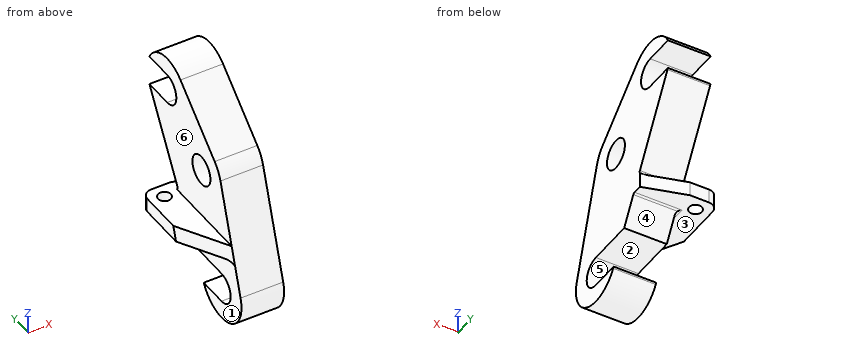
from build123d import *

# Parameters (mm, degrees)
SKETCH1_R                       = 3.15
BOSS_EXTRUDE1_DEPTH             = 9
BOSS_EXTRUDE2_DEPTH             = 6
BOSS_EXTRUDE2_DIRECTION_2_REACH = 244.867
SKETCH3_R                       = 1.35
CUT_EXTRUDE1_DEPTH              = 242.551945874
CHAMFER1_SIZE                   = 6
CHAMFER1_SIZE_2                 = 10
CHAMFER2_SIZE                   = 2.6
CHAMFER2_SIZE2                  = 9
FILLET1_R                       = 2
FILLET2_R                       = 0.5
FILLET3_R                       = 0.5
FILLET4_R                       = 1


with BuildPart() as part:
    # Sketch1 → Boss-Extrude1 (new body)
    with BuildSketch(Plane(origin=(9, 0, 0), x_dir=(0, 0, -1), z_dir=(1, 0, 0))):
        with BuildLine():
            Line((3.523521467, 220.170630859), (3.223774703, 220.343673039))
            Line((3.223774703, 220.343673039), (3.223774703, 214.108306834))
            ThreePointArc((3.223774703, 214.108306834), (0.023774703, 210.908306834), (-3.176225297, 214.108306834))
            Line((-3.176225297, 214.108306834), (-3.176225297, 224.038358312))
            Line((-3.176225297, 224.038358312), (-29.477274378, 239.221811231))
            ThreePointArc((-29.477274378, 239.221811231), (-29.626151265, 239.305353383), (-29.777021142, 239.385240172))
            Line((-29.777021142, 239.385240172), (-29.777021142, 233.159487206))
            ThreePointArc((-29.777021142, 233.159487206), (-32.977021142, 229.959487206), (-36.177021142, 233.159487206))
            Line((-36.177021142, 233.159487206), (-36.177021142, 239.385240172))
            ThreePointArc((-36.177021142, 239.385240172), (-39.85809233, 234.444344903), (-38.208056262, 228.508006627))
            Line((-38.208056262, 228.508006627), (-27.537554982, 216.508006627))
            ThreePointArc((-27.537554982, 216.508006627), (-26.112876869, 215.284825825), (-24.414305812, 214.484366354))
            Line((-24.414305812, 214.484366354), (-2.084011246, 207.433185982))
            ThreePointArc((-2.084011246, 207.433185982), (6.430412997, 211.287848401), (3.523521467, 220.170630859))
        make_face()
        with Locations(Location((-22.306519862, 221.159487206, 0), (0, 0, 180))):
            Circle(SKETCH1_R, mode=Mode.SUBTRACT)
    extrude(amount=-BOSS_EXTRUDE1_DEPTH)

    # Sketch2 → Boss-Extrude2 (add)
    with BuildSketch(Plane.ZY):
        Polygon((8.976225297, 232.108306834), (11.976225297, 232.108306834), (11.976225297, 210.556825276), (8.976225297, 209.609522899), align=None)
    extrude(amount=BOSS_EXTRUDE2_DEPTH)

    # Boss-Extrude2 direction 2: up to this face of the body (flat: up to its plane)
    boss_extrude2_direction_2_end = Plane(part.part.faces().sort_by_distance((9, 222.248813277, 17.342130355))[0])
    # Sketch2 → Boss-Extrude2 direction 2 (add, up to the picked face)
    with BuildSketch(Plane.ZY, mode=Mode.PRIVATE) as boss_extrude2_direction_2_sk1:
        Polygon((8.976225297, 232.108306834), (11.976225297, 232.108306834), (11.976225297, 210.556825276), (8.976225297, 209.609522899), align=None)
    boss_extrude2_direction_2_tool1 = split(extrude(boss_extrude2_direction_2_sk1.sketch, amount=-BOSS_EXTRUDE2_DIRECTION_2_REACH, mode=Mode.PRIVATE), bisect_by=boss_extrude2_direction_2_end, keep=Keep.BOTH, mode=Mode.PRIVATE)
    add(boss_extrude2_direction_2_tool1.solids().sort_by(Axis((0, 221.094043, 10.465473), (1, 0, 0)))[0])

    # Sketch3 → Cut-Extrude1 (cut, through all)
    with BuildSketch(Plane(origin=(0, 0, 8.976225297), x_dir=(-1, 0, 0), z_dir=(0, 0, -1))):
        with Locations(Location((3, 229.108306834, 0), (0, 0, 90))):
            Circle(SKETCH3_R)
    extrude(amount=-CUT_EXTRUDE1_DEPTH, mode=Mode.SUBTRACT)

    # Chamfer1
    # the kernel refuses this chamfer: 10, 6 mm, written as the material it takes off along each edge
    with BuildSketch(Plane(origin=(-6, 218.344374993, 36.638518695), x_dir=(0.9984760801092615, -0.05262494307091041, 0.016617244549774337), z_dir=(0, -0.3011122785042559, -0.9535886931659664))) as chamfer1_piece_1:
        Polygon((CHAMFER1_SIZE * 0.998476080109, -CHAMFER1_SIZE * 0.0551862070598), (-CHAMFER1_SIZE_2 * 0.0551862070598, -CHAMFER1_SIZE_2 * 0.998476080109), (0, 0), align=None)
    extrude(amount=54.8712324, mode=Mode.SUBTRACT)

    # Chamfer2
    chamfer2_edges = [part.edges().sort_by_distance(p)[0] for p in [
        (9, 232.108306834, 10.476225297),
    ]]
    chamfer2_side = [part.faces().sort_by_distance(p)[0] for p in [
        (9, 222.390108053, 17.217310228),
    ]]
    chamfer(chamfer2_edges, length=CHAMFER2_SIZE, length2=CHAMFER2_SIZE2, reference=chamfer2_side[0])

    # Fillet1
    fillet1_edges = [part.edges().sort_by_distance(p)[0] for p in [
        (-6, 232.108306834, 10.476225297),
    ]]
    fillet(fillet1_edges, radius=FILLET1_R)

    # Fillet2
    fillet2_edges = [part.edges().sort_by_distance(p)[0] for p in [
        (4.5, 227.38666684, 8.976225297),
    ]]
    fillet(fillet2_edges, radius=FILLET2_R)

    # Fillet3
    fillet3_edges = [part.edges().sort_by_distance(p)[0] for p in [
        (4.5, 229.118550561, 11.976225297),
    ]]
    fillet(fillet3_edges, radius=FILLET3_R)

    # Fillet4
    fillet4_edges = [part.edges().sort_by_distance(p)[0] for p in [
        (0, 218.642439399, 8.976225297),
    ]]
    fillet(fillet4_edges, radius=FILLET4_R)


solid = part.part
Geometry: final body of the model. Coordinates: model frame, mm. Face numbers are marked on the shaded views. A direction names the side the tool comes from. Give positions to 0.01 mm unless a question says otherwise; leave off trailing zeros. Order: outer loops, then holes, each group sorted by start corner. A loop starts at its lowest first (then second) coordinate and runs counter-clockwise, first axis right, second up. Notation, with made-up numbers: (-27, -1) -> (4, -1) arc R22 cw to (4, 32) -> close; hole circle Ø7 at (60.5, 79). An arc over 180 degrees is marked (long way). Write each question's results on one line, items separated by ' | '.
1) Cut plane D-D (x = 6.25). Output: boundary loops of the cut face in (y, z), and give its area (3 significant figures).
Geometry says:
outline: (207.43, 2.08) arc R7 ccw to (220.17, -3.52) -> (220.34, -3.22) -> (214.11, -3.22) arc R3.2 cw to (214.11, 3.18) -> (224.04, 3.18) -> (227.24, 8.73) arc R0.5 cw to (227.68, 8.98) -> (230.3, 8.98) -> (230.3, 11.98) -> (229.98, 11.98) arc R0.5 cw to (229.55, 12.73) -> (239.22, 29.48) arc R7 ccw to (239.39, 29.78) -> (233.16, 29.78) arc R3.2 cw to (233.16, 36.18) -> (239.39, 36.18) arc R7 ccw to (228.51, 38.21) -> (216.51, 27.54) arc R7 ccw to (214.48, 24.41) -> close; hole circle Ø6.3 at (221.16, 22.31) | area: 641 mm²
2) Set-up query: the marked faces 1, 2 and 3. Return all of +Z, -Z, +X, -X, +Y, -Y with unobstructed straight access to the full face (end or side cutting, diameter ignored); none if empty.
Geometry says:
face 1: -Z, -X, +Y, -Y | face 2: +X, -X, +Y | face 3: -Z, -X, +Y
3) Cut plane B-B (x = 1.5). Output: boundary loops of the cut face in (y, z).
Geometry says:
outline: (207.43, 2.08) arc R7 ccw to (220.17, -3.52) -> (220.34, -3.22) -> (214.11, -3.22) arc R3.2 cw to (214.11, 3.18) -> (224.04, 3.18) -> (227.24, 8.73) arc R0.5 cw to (227.68, 8.98) -> (231.67, 8.98) -> (231.67, 11.98) -> (229.98, 11.98) arc R0.5 cw to (229.55, 12.73) -> (239.22, 29.48) arc R7 ccw to (239.39, 29.78) -> (233.16, 29.78) arc R3.2 cw to (233.16, 36.18) -> (239.39, 36.18) arc R7 ccw to (228.51, 38.21) -> (216.51, 27.54) arc R7 ccw to (214.48, 24.41) -> close; hole circle Ø6.3 at (221.16, 22.31)
4) Draft query along Z for the marked faces 4, 5 and 6. Return one class per face: released by +Z, released by -Z, zero draft, split by the parting line, or undercut.
Geometry says:
face 4: released by -Z | face 5: undercut | face 6: zero draft
5) Cut plane C-C (x = -3). Output: boundary loops of the cut face in (y, z).
Geometry says:
outline: (214.85, 8.98) -> (227.76, 8.98) -> (227.76, 11.98) -> (215.8, 11.98) -> close; (230.46, 8.98) -> (232.11, 8.98) -> (232.11, 11.98) -> (230.46, 11.98) -> close
6) First-contact query: pin 1 Ø6 at (x, y) = (2.5, 217) entering from +Z; pin 2 Ø4 at (y, z) = (221.16, 22.31) entering from +X; pin 3 Ø2.5 at (x, z) = (-3, 11) entering from +Y; pin 4 Ø4.5 at (x, y) = (2.5, 218.5) entering from -Z. Flat tips, straight axial feed; report the tip coordinate or a pass-through.
Geometry says:
pin 1: stops at z = 30.64 | pin 2: passes through | pin 3: stops at y = 232.11 | pin 4: stops at z = -6.69
7) Cut plane A-A (y = 223.5). Output: boundary loops of the cut face in (x, z), and give its area (3 significant figures).
Geometry says:
outline: (-6, 8.98) -> (-1, 8.98) arc R1 cw to (0, 7.98) -> (0, 3.18) -> (9, 3.18) -> (9, 20.2) -> (0, 20.2) -> (0, 11.98) -> (-6, 11.98) -> close; (0, 24.41) -> (9, 24.41) -> (9, 33.75) -> (0, 33.75) -> close | area: 255 mm²
8) Line query: line 1 along X through (y, z) = (220.5, 6); line 2 along Z through (x, y) = (5.5, 233.5); line 3 along Z through (x, y) = (-0.25, 229). Output: solid intervals per line, ascending.
Geometry says:
line 1: x = 0 to 9 | line 2: z = 19.57 to 29.78, 36.18 to 39.97 | line 3: z = 8.98 to 11.98
